The listing builds one solid part. Answer for the finished solid, in the listing's coordinates (mm). Round coordinates to 2 decimals unless told otherwise and drop trailing zeros. Loops run counter-clockwise (first coordinate to the right, second up) from the corner with the lowest first, then second, coordinate; pieces in that order, holes last. Notation, with made-up numbers: (-21, -4) -> (-17, -4) arc R19 cw to (-17, 31) -> close; hole circle Ø10 at (-18, 25). An arc over 180 degrees is marked (long way). Answer in a Markdown table with one row per item. Add a question column.
```python
from build123d import *

# Parameters (mm, degrees)
SKETCH1_R           = 2.1828125
SKETCH1_R_2         = 2.38125
BOSS_EXTRUDE1_DEPTH = 1.5875


with BuildPart() as part:
    # Sketch1 → Boss-Extrude1 (new body)
    with BuildSketch(Plane(origin=(0, 0, 0), x_dir=(1, 0, 0), z_dir=(0, 1, 0))):
        with BuildLine():
            Line((-76.2, -19.05), (76.2, -19.05))
            ThreePointArc((76.2, -19.05), (79.801136223, -17.930135553), (82.132104124, -14.965533197))
            Line((82.132104124, -14.965533197), (91.194236912, 8.762883297))
            ThreePointArc((91.194236912, 8.762883297), (91.521572666, 9.959813472), (91.609879929, 11.197550265))
            Line((91.609879929, 11.197550265), (89.542716066, 88.780125789))
            ThreePointArc((89.542716066, 88.780125789), (88.21446111, 92.500361917), (84.943711156, 94.715449457))
            Line((84.943711156, 94.715449457), (60.525881406, 101.710418382))
            ThreePointArc((60.525881406, 101.710418382), (55.697183415, 101.159011684), (52.672681737, 97.354703175))
            ThreePointArc((52.672681737, 97.354703175), (31.779047976, 62.743000168), (-3.710967925, 43.378788638))
            Line((-3.710967925, 43.378788638), (-54.689770483, 39.419061875))
            ThreePointArc((-54.689770483, 39.419061875), (-56.360545493, 39.058557607), (-57.874640982, 38.265483014))
            Line((-57.874640982, 38.265483014), (-88.938751905, 16.205768315))
            ThreePointArc((-88.938751905, 16.205768315), (-91.339222957, 12.870012291), (-91.194236912, 8.762883297))
            Line((-91.194236912, 8.762883297), (-82.132104124, -14.965533197))
            ThreePointArc((-82.132104124, -14.965533197), (-79.801136223, -17.930135553), (-76.2, -19.05))
        make_face()
        with Locations(Location((0, 0, 0), (0, 0, 270))):
            Circle(SKETCH1_R, mode=Mode.SUBTRACT)
        with Locations(Location((12.7, 0, 0), (0, 0, 270))):
            Circle(SKETCH1_R_2, mode=Mode.SUBTRACT)
        with Locations(Location((25.4, 0, 0), (0, 0, 270))):
            Circle(SKETCH1_R_2, mode=Mode.SUBTRACT)
        with Locations(Location((-38.1, -12.7, 0), (0, 0, 270))):
            Circle(SKETCH1_R, mode=Mode.SUBTRACT)
        with Locations(Location((-50.8, -12.7, 0), (0, 0, 270))):
            Circle(SKETCH1_R, mode=Mode.SUBTRACT)
        with Locations(Location((-63.5, -12.7, 0), (0, 0, 270))):
            Circle(SKETCH1_R, mode=Mode.SUBTRACT)
        with Locations(Location((-76.2, -12.7, 0), (0, 0, 270))):
            Circle(SKETCH1_R, mode=Mode.SUBTRACT)
        with Locations(Location((38.1, -12.7, 0), (0, 0, 270))):
            Circle(SKETCH1_R, mode=Mode.SUBTRACT)
        with Locations(Location((50.8, -12.7, 0), (0, 0, 270))):
            Circle(SKETCH1_R, mode=Mode.SUBTRACT)
        with Locations(Location((63.5, -12.7, 0), (0, 0, 270))):
            Circle(SKETCH1_R, mode=Mode.SUBTRACT)
        with Locations(Location((76.2, -12.7, 0), (0, 0, 270))):
            Circle(SKETCH1_R, mode=Mode.SUBTRACT)
        with Locations(Location((-54.198021866, 33.088131193, 0), (0, 0, 270))):
            Circle(SKETCH1_R, mode=Mode.SUBTRACT)
        with Locations(Location((54.198021866, 33.088131193, 0), (0, 0, 270))):
            Circle(SKETCH1_R, mode=Mode.SUBTRACT)
        with Locations(Location((-85.262132788, 11.028416494, 0), (0, 0, 270))):
            Circle(SKETCH1_R, mode=Mode.SUBTRACT)
        with Locations(Location((85.262132788, 11.028416494, 0), (0, 0, 270))):
            Circle(SKETCH1_R, mode=Mode.SUBTRACT)
        with Locations(Location((0, 38.1, 0), (0, 0, 270))):
            Circle(SKETCH1_R, mode=Mode.SUBTRACT)
        with Locations(Location((12.646044992, 36.930578751, 0), (0, 0, 270))):
            Circle(SKETCH1_R, mode=Mode.SUBTRACT)
        with Locations(Location((-12.646044992, 36.930578751, 0), (0, 0, 270))):
            Circle(SKETCH1_R, mode=Mode.SUBTRACT)
        with Locations(Location((41.551976873, 34.257552442, 0), (0, 0, 270))):
            Circle(SKETCH1_R_2, mode=Mode.SUBTRACT)
        with Locations(Location((28.905931881, 35.426973691, 0), (0, 0, 270))):
            Circle(SKETCH1_R_2, mode=Mode.SUBTRACT)
        with Locations(Location((76.2, 64.193162268, 0), (0, 0, 270))):
            Circle(SKETCH1_R, mode=Mode.SUBTRACT)
        with Locations(Location((51.782170249, 71.188131193, 0), (0, 0, 270))):
            Circle(SKETCH1_R_2, mode=Mode.SUBTRACT)
        with Locations(Location((63.991085125, 67.690646731, 0), (0, 0, 270))):
            Circle(SKETCH1_R_2, mode=Mode.SUBTRACT)
        with Locations(Location((-41.551976873, 34.257552442, 0), (0, 0, 270))):
            Circle(SKETCH1_R, mode=Mode.SUBTRACT)
        with Locations(Location((-28.905931881, 35.426973691, 0), (0, 0, 270))):
            Circle(SKETCH1_R, mode=Mode.SUBTRACT)
        with Locations(Location((58.777139174, 95.605960944, 0), (0, 0, 270))):
            Circle(SKETCH1_R, mode=Mode.SUBTRACT)
        with Locations(Location((83.194968925, 88.610992019, 0), (0, 0, 270))):
            Circle(SKETCH1_R, mode=Mode.SUBTRACT)
    extrude(amount=BOSS_EXTRUDE1_DEPTH)


solid = part.part
```
Item 1: Section D-D, the plane z = -76.5 is taken. Write down the section's boundary in (x, y).
Item 2: Section B-B, the plane y = 0.65 is taken. Give the number of separate pieces and of enclosed holes in the cut face, and give its area (3 significant figures).
Item 3: Consider L1, parallel to X at y = 1.1, z = -69.5; L2, parallel to Z at x = 62.5, y = 1.2; L3, parallel to Z at x = -54.5, y = 1.15. Determine where each line is inside the solid, lowest interval first. Write a range as from..to.
Item 4: The mould has two halves that part along X. Classify faces 1 (the cylindrical face through (79.76, 0.78, 17.96)), 2 (the cylindrical face through (-55.526, 0.783, -34.82)), 3 (the flat face through (-86.727, 0.783, 2.935)): +X half, -X half, draft (parallel to the pull), parting line (faces both ways), or undercut.
Item 5: Section A-A, the plane x = 0 is taken. Write down the section's boundary in (y, z).
Item 6: Section C-C, the plane z = -56.5 is taken. Write down the section's boundary in (x, y), and give its area (3 significant figures).
Here are the results:
| question | item | result |
|---|---|---|
| 1 | outline | (43.17, 0) -> (89.87, 0) -> (89.87, 1.59) -> (43.17, 1.59) -> close |
| 2 | separate pieces | 1 |
| 2 | enclosed holes | 27 |
| 2 | area | 13,000 mm² |
| 3 | L1 | x = 38.04..50.1, 53.46..62.44, 65.54..90.06 |
| 3 | L2 | z = -101.14..-69.55, -65.83..10.76, 14.64..19.05 |
| 3 | L3 | z = -39.43..-35.25, -30.93..19.05 |
| 4 | face 1 | +X half |
| 4 | face 2 | undercut |
| 4 | face 3 | -X half |
| 5 | outline | (0, -44.37) -> (1.59, -44.37) -> (1.59, -40.28) -> (0, -40.28) -> close; (0, -35.92) -> (1.59, -35.92) -> (1.59, -2.18) -> (0, -2.18) -> close; (0, 2.18) -> (1.59, 2.18) -> (1.59, 19.05) -> (0, 19.05) -> close |
| 6 | outline | (24.38, 0) -> (90.4, 0) -> (90.4, 1.59) -> (24.38, 1.59) -> close |
| 6 | area | 105 mm² |
